from build123d import *

# Parameters (mm, degrees)
BOSS_EXTRU_1_DEPTH      = 11.8
ESQUISSE2_R             = 5.9
BOSS_EXTRU_3_DEPTH      = 4
ESQUISSE3_R             = 2.5
BOSS_EXTRU_4_DEPTH      = 4
ESQUISSE5_R             = 2.3
BOSS_EXTRU_5_DEPTH      = 3.63
ENL_V_MAT_EXTRU_7_REACH = 20.4
ESQUISSE16_W            = 3.6
ESQUISSE16_H            = 1.2
BOSS_EXTRU_8_DEPTH      = 1.2


with BuildPart() as part:
    # Esquisse1 → Boss.-Extru.1 (new body)
    with BuildSketch(Plane.XY):
        Polygon((0, 0), (-22.5, 0), (-22.5, 15.9), (-27.2, 15.9), (-27.2, 18.4), (-22.5, 18.4), (-22.5, 22.7), (0, 22.7), (0, 18.4), (4.7, 18.4), (4.7, 15.9), (0, 15.9), align=None)
    extrude(amount=BOSS_EXTRU_1_DEPTH)

    # Esquisse2 → Boss.-Extru.3 (add)
    with BuildSketch(Plane(origin=(0, 22.7, 0), x_dir=(1, 0, 0), z_dir=(0, 1, 0))):
        with Locations((-16.6, -5.9)):
            Circle(ESQUISSE2_R)
    extrude(amount=BOSS_EXTRU_3_DEPTH)

    # Esquisse3 → Boss.-Extru.4 (add)
    with BuildSketch(Plane(origin=(0, 22.7, 0), x_dir=(1, 0, 0), z_dir=(0, 1, 0))):
        with Locations((-10.3, -5.738368037)):
            Circle(ESQUISSE3_R)
    extrude(amount=BOSS_EXTRU_4_DEPTH)

    # Esquisse5 → Boss.-Extru.5 (add)
    with BuildSketch(Plane(origin=(0, 26.7, 0), x_dir=(1, 0, 0), z_dir=(0, 1, 0))):
        with Locations((-16.6, -5.9)):
            Circle(ESQUISSE5_R)
    extrude(amount=BOSS_EXTRU_5_DEPTH)

    # Esquisse6 → Enlèv. mat.-Extru.7 (cut, up to next)
    with BuildSketch(Plane(origin=(0, 18.4, 0), x_dir=(1, 0, 0), z_dir=(0, 1, 0)), mode=Mode.PRIVATE) as enl_v_mat_extru_7_sk1:
        with BuildLine():
            Line((6.661887407, -5.9), (6.661887407, -5.25))
            Line((6.661887407, -5.25), (3.159934208, -5.25))
            ThreePointArc((3.159934208, -5.25), (1.4, -5.9), (3.159934208, -6.55))
            Line((3.159934208, -6.55), (6.661887407, -6.55))
            Line((6.661887407, -6.55), (6.661887407, -5.9))
        make_face()
    enl_v_mat_extru_7_tool1 = extrude(enl_v_mat_extru_7_sk1.sketch, amount=-ENL_V_MAT_EXTRU_7_REACH, mode=Mode.PRIVATE) & part.part
    add(enl_v_mat_extru_7_tool1.solids().sort_by_distance((3.903633, 18.4, 5.9))[0], mode=Mode.SUBTRACT)
    # Esquisse6 → Enlèv. mat.-Extru.7 (cut, up to next)
    with BuildSketch(Plane(origin=(0, 18.4, 0), x_dir=(1, 0, 0), z_dir=(0, 1, 0)), mode=Mode.PRIVATE) as enl_v_mat_extru_7_sk2:
        with BuildLine():
            Line((-29.161887407, -5.25), (-25.659934208, -5.25))
            ThreePointArc((-25.659934208, -5.25), (-23.9, -5.9), (-25.659934208, -6.55))
            Line((-25.659934208, -6.55), (-29.161887407, -6.55))
            Line((-29.161887407, -6.55), (-29.161887407, -5.9))
            Line((-29.161887407, -5.9), (-29.161887407, -5.25))
        make_face()
    enl_v_mat_extru_7_tool2 = extrude(enl_v_mat_extru_7_sk2.sketch, amount=-ENL_V_MAT_EXTRU_7_REACH, mode=Mode.PRIVATE) & part.part
    add(enl_v_mat_extru_7_tool2.solids().sort_by_distance((-26.403633, 18.4, 5.9))[0], mode=Mode.SUBTRACT)

    # Esquisse16 → Boss.-Extru.8 (add)
    with BuildSketch(Plane.ZY.offset(22.5)):
        with Locations((5.9, 5.1)):
            Rectangle(ESQUISSE16_W, ESQUISSE16_H)
    extrude(amount=BOSS_EXTRU_8_DEPTH)


solid = part.part
Read the model definition and answer for the solid it produces. Units are mm, in the model's axes. A direction names the side the tool comes from. Give positions to 0.01 mm unless a question says otherwise; leave off trailing zeros. Loops run counter-clockwise (first coordinate to the right, second up) from the corner with the lowest first, then second, coordinate; pieces in that order, holes last. Notation, with made-up numbers: (81.5, 68) - (85.5, 68) arc R9 cw to (85.5, 78) - close; hole circle Ø3 at (14.25, 82.5). An arc over 180 degrees is marked (long way). Answer as CSV lines item,"result". Start each with the question number.
1) Which of the six approach directions +Z, -Z, +X, -X, +Y, -Y give full straight-line access (tool end or side, diameter ignored) to faces 4 (the face through (4, 17, 6.55)), 5 (the face through (1, 15.9, 6)), 6 (the face through (-14, 26.7, 6))?
2) Find section C-C (z = 1.75). Write down the section's boundary in (x, y).
3) Straight lines are drawn through the part: L1, parallel to Z at x = 2.4, y = 16.8; L2, parallel to Y at x = -14.5, z = 0.75; L3, parallel to X at y = 12, z = 3.5. For each, find the intervals that lie inside material, in ascending order. Write a range as from..to.
4) Find section D-D (y = 12). Write down the section's boundary in (x, z).
5) Each of these flat-tipped pins is pushed along its axis until it touches: pin 1 Ø2 at (x, z) = (-19, 10.5) entering from +Y; pin 2 Ø1.3 at (y, z) = (5, 6.5) entering from -X; pin 3 Ø6 at (y, z) = (7, 8.5) entering from +X. Where does it stop, or does it pass through?
6) Determine the mould class of faces 1 (the face through (-26, 17, 5.25)), 2 (the face through (4.7, 17, 9)), 3 (the face through (-23, 5, 7.7)) for opening direction Z: released by +Z, released by -Z, zero draft, split by the parting line, or undercut.
7) Find section B-B (x = 2.4). Write down the section's boundary in (y, z).
8) Find section A-A (x = -23). Write down the section's boundary in (y, z).
Findings below:
1,face 4,"+X, +Y, -Y"
1,face 5,"+Z, -Z, +X, -Y"
1,face 6,"+Y"
2,outline,"(-27.2, 15.9) - (-22.5, 15.9) - (-22.5, 0) - (0, 0) - (0, 15.9) - (4.7, 15.9) - (4.7, 18.4) - (0, 18.4) - (0, 22.7) - (-12.41, 22.7) - (-12.41, 26.7) - (-20.79, 26.7) - (-20.79, 22.7) - (-22.5, 22.7) - (-22.5, 18.4) - (-27.2, 18.4) - close"
3,L1,"0..4.9, 6.9..11.8"
3,L2,"0..26.7"
3,L3,"-22.5..0"
4,outline,"(-22.5, 0) - (0, 0) - (0, 11.8) - (-22.5, 11.8) - close"
5,pin 1,"y = 26.7"
5,pin 2,"x = -23.7"
5,pin 3,"x = 0"
6,face 1,"undercut"
6,face 2,"zero draft"
6,face 3,"released by +Z"
7,outline,"(15.9, 0) - (18.4, 0) - (18.4, 4.9) - (15.9, 4.9) - close; (15.9, 6.9) - (18.4, 6.9) - (18.4, 11.8) - (15.9, 11.8) - close"
8,outline,"(4.5, 4.1) - (5.7, 4.1) - (5.7, 7.7) - (4.5, 7.7) - close; (15.9, 0) - (18.4, 0) - (18.4, 11.8) - (15.9, 11.8) - close"
